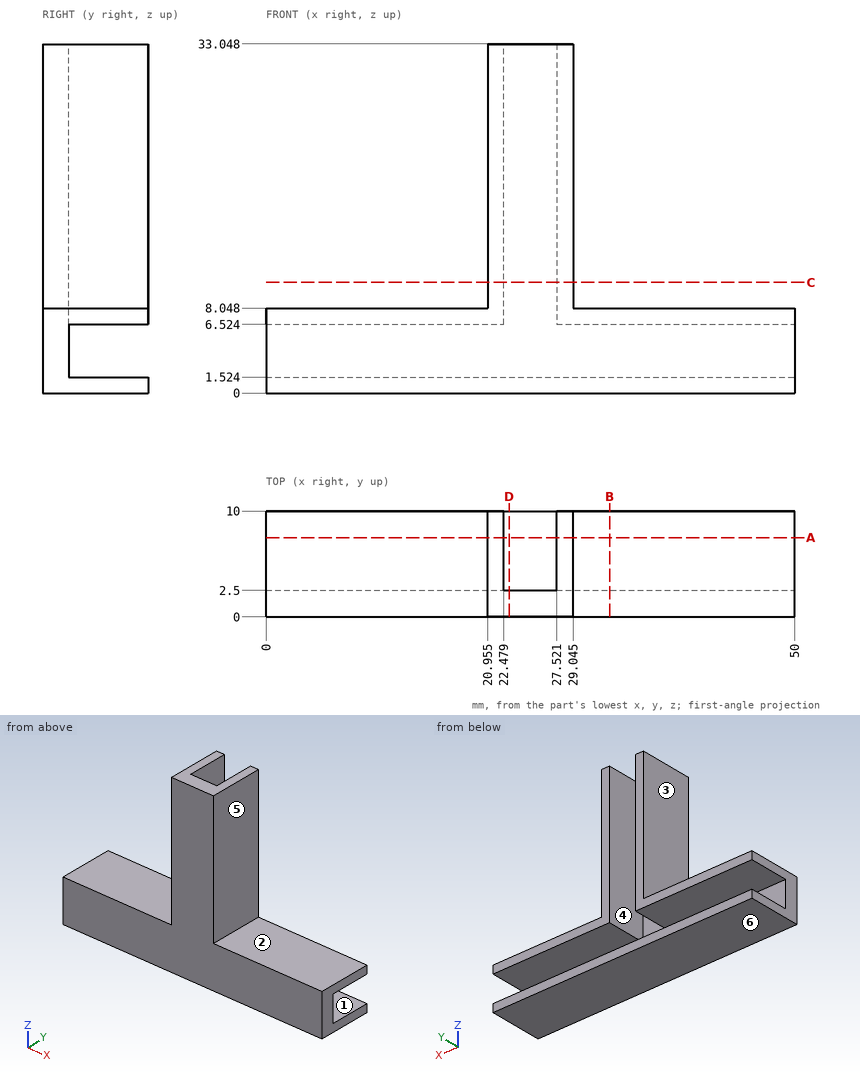
Study the drawing (mm; zero at the part's minimum x, y, z) and answer. A direction names the side the tool comes from. Round coordinates to 2 decimals unless told otherwise and drop trailing zeros. Loops run counter-clockwise (first coordinate to the right, second up) from the corner with the lowest first, then second, coordinate; pieces in that order, holes last.
Q1. For a pull along X with two mould halves and no side action, classify the marked faces 4, 5 and 6 as released by +X, released by -X, zero draft, split by the parting line, or undercut.
Q2. Given pin 1 Ø3 at (y, z) = (6.5, 21) entering from +X (3 decimals); pin 2 Ø5 at (x, y) = (36, 5) entering from +Z; pin 3 Ø4 at (y, z) = (7.5, 20.5) entering from -X (3 decimals), each flat-ended and moving along its own axis, determine where each tip first touches the part or whether it passes through.
Q3. Section D-D, the plane x = 23 is taken. Determine the outline of the cut face in (y, z).
Q4. Section A-A, the plane y = 7.5 is taken. Determine the outline of the cut face in (x, z) (3 decimals).
Q5. Which of the six approach directions +Z, -Z, +X, -X, +Y, -Y give full straight-line access (tool end or side, diameter ignored) to the marked faces 1, 2 and 3?
Q6. Find the intervals of material crossed by line 1 (X direction, y = 3.75, z = 15) (3 decimals); line 2 (Z direction, x = 47.5, y = 8); line 3 (Y direction, x = 18, z = 4), in increasing order.
Q7. Section B-B, the plane x = 32.5 is taken. Determine the outline of the cut face in (y, z).
Q8. Section C-C, the plane z = 10.5 is taken. Determine the outline of the cut face in (x, y) (3 decimals).
Completed:
1. face 4: undercut
1. face 5: released by +X
1. face 6: zero draft
2. pin 1: stops at x = 29.045
2. pin 2: stops at z = 8.05
2. pin 3: stops at x = 20.955
3. outline: (0, 0) - (10, 0) - (10, 1.52) - (2.5, 1.52) - (2.5, 33.05) - (0, 33.05) - close
4. outline: (0, 0) - (50, 0) - (50, 1.524) - (0, 1.524) - close; (0, 6.524) - (22.479, 6.524) - (22.479, 33.048) - (20.955, 33.048) - (20.955, 8.048) - (0, 8.048) - close; (27.521, 6.524) - (50, 6.524) - (50, 8.048) - (29.045, 8.048) - (29.045, 33.048) - (27.521, 33.048) - close
5. face 1: +X, -X, +Y
5. face 2: +Z, +X, +Y, -Y
5. face 3: +Z, -X, +Y, -Y
6. line 1: x = 20.955 to 22.479, 27.521 to 29.045
6. line 2: z = 0 to 1.52, 6.52 to 8.05
6. line 3: y = 0 to 2.5
7. outline: (0, 0) - (10, 0) - (10, 1.52) - (2.5, 1.52) - (2.5, 6.52) - (10, 6.52) - (10, 8.05) - (0, 8.05) - close
8. outline: (20.955, 0) - (29.045, 0) - (29.045, 10) - (27.521, 10) - (27.521, 2.5) - (22.479, 2.5) - (22.479, 10) - (20.955, 10) - close
